Check sheet for the modelled part. Datum: model origin and axes. Units: mm. A direction names the side the tool comes from. Round coordinates to 2 decimals unless told otherwise and drop trailing zeros. Write each loop counter-clockwise with the first axis right and the second up, starting at its lowest first coordinate (ties: lowest second). Pieces come first, ordered by that corner, then holes. Notation, with made-up numbers: (67, -36) -> (96, -36) arc R15 cw to (96, -32) -> close; hole circle Ø2 at (-37, -35.5). An arc over 180 degrees is marked (long way). One line per item, written item: value.
from build123d import *

# Parameters (mm, degrees)
BOSS_EXTRU_2_DEPTH           = 5
BOSS_EXTRU_8_START           = -1
BOSS_EXTRU_8_DEPTH           = 5
ENL_V_MAT_EXTRU_3_DEPTH      = 57.886804216
ENL_V_MAT_EXTRU_3_DEPTH_BACK = 57.886804216
ESQUISSE8_OUTSIDE_W          = 48.282
ESQUISSE8_OUTSIDE_H          = 25.106


with BuildPart() as part:
    # Esquisse1 → Boss.-Extru.2 (new body)
    with BuildSketch(Plane.XY):
        with BuildLine():
            ThreePointArc((5.586871342, -2.187891362), (5.144080872, -3.088435199), (4.557392942, -3.902584986))
            ThreePointArc((4.557392942, -3.902584986), (-5.144080872, 3.088435199), (5.586871342, -2.187891362))
        make_face()
    extrude(amount=BOSS_EXTRU_2_DEPTH)

    # Esquisse7 → Boss.-Extru.8 (add, symmetric)
    with BuildSketch(Plane(origin=(0, 0, 0), x_dir=(-1, 0, 0), z_dir=(0, 0, -1)).offset(BOSS_EXTRU_8_START)):
        with BuildLine():
            Line((23.267356356, 49.614121246), (13.267356356, 49.614121246))
            Line((13.267356356, 49.614121246), (14.157356645, 44.566678785))
            Line((14.157356645, 44.566678785), (20.047511648, 44.566678785))
            ThreePointArc((20.047511648, 44.566678785), (19.869115778, 21.373460498), (3.835346807, 4.614121246))
            ThreePointArc((3.835346807, 4.614121246), (5.409269967, 2.596112175), (5.999067404, 0.105784144))
            ThreePointArc((5.999067404, 0.105784144), (25.143375104, 21.19405426), (23.267356356, 49.614121246))
        make_face()
    extrude(amount=BOSS_EXTRU_8_DEPTH, both=True)

    # Esquisse8 outside → Enlèv. mat.-Extru.3 (cut, two sides: drawn at the far end of the back side and taken through both)
    with BuildSketch(Plane(origin=(0, 0, 0), x_dir=(1, 0, 0), z_dir=(0, 1, 0)).offset(-ENL_V_MAT_EXTRU_3_DEPTH_BACK)):
        with Locations((-10.588, -1)):
            Rectangle(ESQUISSE8_OUTSIDE_W, ESQUISSE8_OUTSIDE_H)
        Polygon((-31.025150446, 0), (-31.025150446, -5), (-4.47625447, -5), (6.185645272, -5), (6.185645272, 0), (-4.47625447, 0), align=None, mode=Mode.SUBTRACT)
    extrude(amount=ENL_V_MAT_EXTRU_3_DEPTH + ENL_V_MAT_EXTRU_3_DEPTH_BACK, mode=Mode.SUBTRACT)


solid = part.part
Item 1: Sectioned sample at B-B (z = 2.4). Enter the section's corners in (x, y), then the cut area to 3 significant figures.
Result set:
outline: (-23.27, 49.61) arc R36.44 ccw to (-6, 0.11) arc R6 ccw (long way) to (-3.84, 4.61) arc R31.44 cw to (-20.05, 44.57) -> (-14.16, 44.57) -> (-13.27, 49.61) -> close
area: 417 mm^2
Item 2: Sectioned sample at C-C (x = 2). Enter the section's corners in (y, z), then the cut area to 3 significant figures.
Result set:
outline: (-5.66, 0) -> (5.66, 0) -> (5.66, 5) -> (-5.66, 5) -> close
area: 56.6 mm^2
Item 3: Depth check by flat-ended pin: pin 1 (3 mm diameter, centred on x = -20, z = 1, fed in from -Y); pin 2 (3 mm diameter, centred on x = -9.5, z = 0.5, fed in from -Y); pin 3 (1 mm diameter, centred on y = 12, z = 2, fed in from -X). Enter the tip coordinate at first touch or a pass-through.
Result set:
pin 1: y = 9.59
pin 2: y = 1.1
pin 3: x = -20.73
Item 4: Release check for a two-part mould opening along Y. For faces 3 (the flat face through (-18, 49.614, 2)), 4 (the cylindrical face through (-25.006, 20.808, 2.465)), 5 (the flat face through (-17, 15, 0)), 6 (the flat face through (-17, 44.567, 2)) record: pulls with the +Y half, pulls with the -Y half, needs draft (parallel to the pull), parting line crosses it, or undercut.
Result set:
face 3: pulls with the +Y half
face 4: parting line crosses it
face 5: needs draft
face 6: undercut
Item 5: Tool access check on faces 1 (the flat face through (-18, 15, 5)), 2 (the flat face through (-13.706, 47.126, 2.465)). Record the directions out of +Z, -Z, +X, -X, +Y, -Y that give a thin tool (end or side, any length) a straight path to the whole face; none if there is none.
Result set:
face 1: +Z, +X, -X, +Y, -Y
face 2: +Z, -Z, +X
Item 6: Sectioned sample at A-A (x = -19). Enter the section's corners in (y, z).
Result set:
outline: (10.19, 0) -> (19.42, 0) -> (19.42, 5) -> (10.19, 5) -> close; (44.57, 0) -> (49.61, 0) -> (49.61, 5) -> (44.57, 5) -> close
Item 7: Sectioned sample at D-D (y = 17). Enter the section's corners in (x, z), then the cut area to 3 significant figures.
Result set:
outline: (-23.38, 0) -> (-17.68, 0) -> (-17.68, 5) -> (-23.38, 5) -> close
area: 28.5 mm^2
Item 8: Material ranges on line 1 along Y through (x, z) = (-17, 0.5); line 2 along Y through (x, z) = (-19, 1.65); line 3 along X through (y, z) = (5.5, 2.75), recorded low to high.
Result set:
line 1: 7.93 to 15.91, 44.57 to 49.61
line 2: 10.19 to 19.42, 44.57 to 49.61
line 3: -14.42 to -5.62, -2.4 to 2.4
